Input: dimensioned drawing with shaded views. Units: mm. Origin: part minimum x, y, z. A direction names the side the tool comes from. Coordinates: 2 decimals unless noted, no trailing zeros. Order: outer loops, then holes, each group sorted by start corner. A loop starts at its lowest first (then second) coordinate and runs counter-clockwise, first axis right, second up.
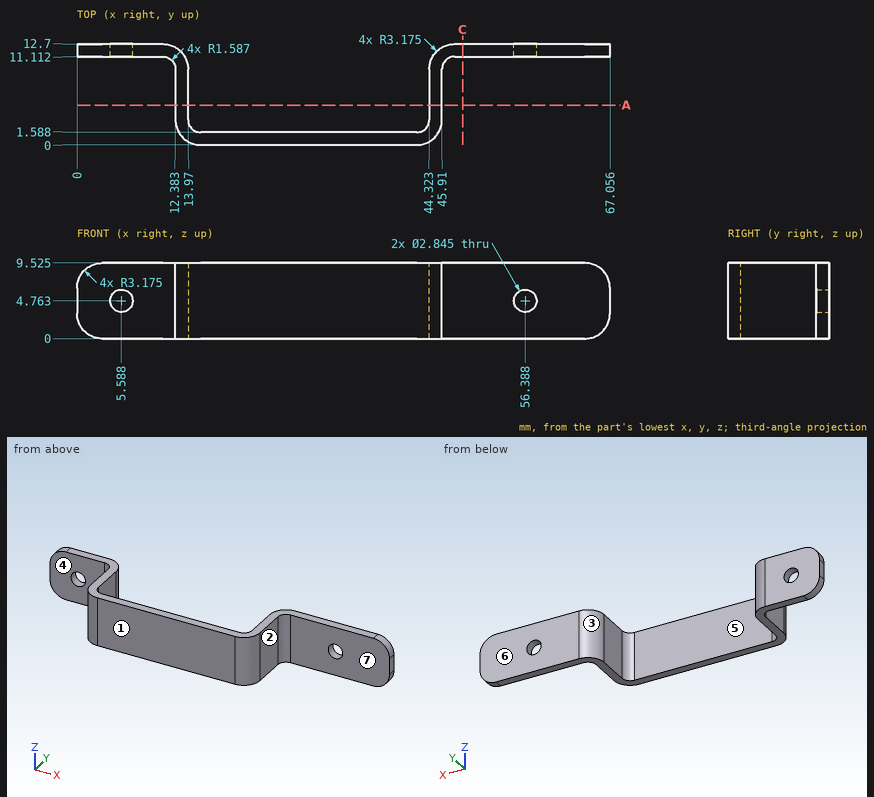
1. Section query A-A on y = 5. Return loops of the section in (x, z) (1 decimal).
Findings:
outline: (12.4, 0) - (14, 0) - (14, 9.5) - (12.4, 9.5) - close; (44.3, 0) - (45.9, 0) - (45.9, 9.5) - (44.3, 9.5) - close
2. Pin query (flat end, axial travel): P1, Ø3, axis at x = 60.5, z = 3.5, coming from the -Y side; P2, Ø2, axis at x = 46.5, y = 5.5, coming from the +Z side (1 decimal); P3, Ø5, axis at y = 6.5, z = 7, coming from the +X side; P4, Ø2.5, axis at x = 56.39, z = 4.76, coming from the +Y side (3 decimals). Return the tip coordinate at first contact, or that it passes through.
Findings:
P1: stops at y = 11.11
P2: stops at z = 9.5
P3: stops at x = 45.91
P4: passes through
3. Draft query along X for the marked faces 1, 2 and 3. Return one class per face: released by +X, released by -X, zero draft, split by the parting line, or undercut.
Findings:
face 1: zero draft
face 2: released by +X
face 3: undercut
4. Ray query, line 1 (X direction, y = 5.75, z = 3.5); line 2 (X direction, y = 11.25, z = 4) (1 decimal); line 3 (Y direction, x = 23, z = 4.75). Return the intervals inside material, ascending.
Findings:
line 1: x = 12.38 to 13.97, 44.32 to 45.91
line 2: x = 0 to 4.4, 6.8 to 13.5, 44.8 to 55.2, 57.6 to 67.1
line 3: y = 0 to 1.59
5. Section query C-C on x = 48.5. Return loops of the section in (y, z) (1 decimal).
Findings:
outline: (11.1, 0) - (12.7, 0) - (12.7, 9.5) - (11.1, 9.5) - close
6. Access query for the marked faces 4, 5, 6 and 7. Directions: +Z, -Z, +X, -X, +Y, -Y. A direction counts if a zero-diameter tool reaches every point of the face in a straight line with its end or side. Return the directions, or none.
Findings:
face 4: +Z, -Z, -X, -Y
face 5: +Z, -Z, +Y
face 6: +Z, -Z, +X, -X, +Y
face 7: +Z, -Z, +X, -Y
